For this review, use the dimensioned drawing (mm, ordinates from the lowest corner) and the shaded views. A direction names the side the tool comes from. Coordinates: 2 decimals unless noted, no trailing zeros. Order: outer loops, then holes, each group sorted by start corner. A loop starts at its lowest first (then second) coordinate and runs counter-clockwise, first axis right, second up. Notation, with made-up numbers: M 6.5,13 L 25.5,13 A37 cw 25.5,50 Z; hole C 66.5,-1.5 d5. An arc over 180 degrees is marked long. Answer in a Markdown table with one row per item.
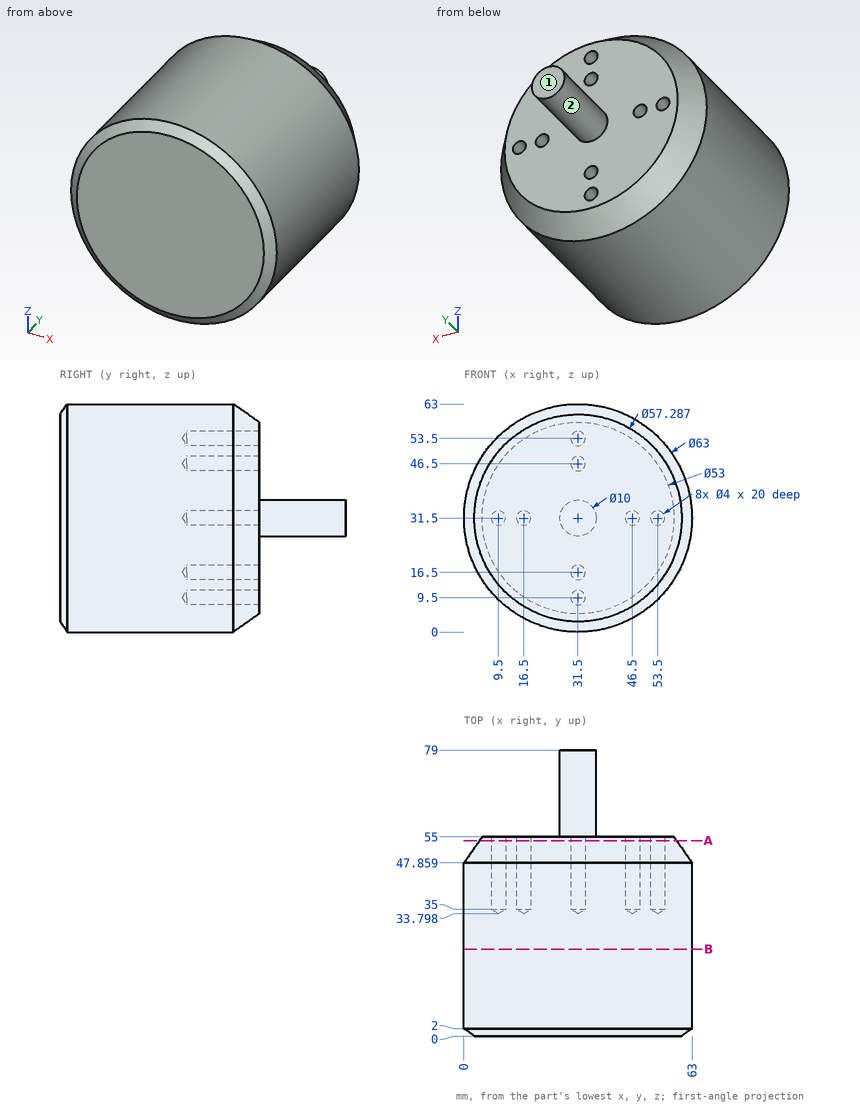
(1) Insertion check: P1, Ø12, axis at x = 24, y = 26.5, coming from the +Z side; P2, Ø1, axis at x = 8.5, y = 35.5, coming from the +Z side (1 decimal); P3, Ø3, axis at x = 45, y = 47, coming from the -Z side (1 decimal). Each pin has a flat end and moves straight along its axis. Give the tip position at first contact, or say it passes through.
Report:
| item | result |
|---|---|
| P1 | z = 62.96 |
| P2 | z = 53.5 |
| P3 | z = 2.4 |
(2) To check wall thickness, follow line 1 (X direction, y = 43, z = 31.5); line 2 (X direction, y = 47, z = 31) (1 decimal). State the ranges of each line that lie inside material, in increasing order. Write a range as [from, to].
Report:
| item | result |
|---|---|
| line 1 | [0, 7.5], [11.5, 14.5], [18.5, 44.5], [48.5, 51.5], [55.5, 63] |
| line 2 | [0, 7.6], [11.4, 14.6], [18.4, 44.6], [48.4, 51.6], [55.4, 63] |
(3) Take a section at B-B (y = 24). Write out the cut boundary in (x, z), then the cut area to 3 significant figures.
Report:
| item | result |
|---|---|
| outline | C 31.5,31.5 d63 |
| area | 3,120 mm^2 |
(4) Machinability: for the marked faces 1 and 2, which of the approach directions +Z, -Z, +X, -X, +Y, -Y give a long, thin tool a straight path to every point of the face, cutting with its end or side? Answer none if there is none.
Report:
| item | result |
|---|---|
| face 1 | +Z, -Z, +X, -X, +Y |
| face 2 | +Y |
(5) Take a section at A-A (y = 54). State how many separate pieces and enclosed holes the cut face has, then the cut area to 3 significant figures.
Report:
| item | result |
|---|---|
| separate pieces | 1 |
| enclosed holes | 8 |
| area | 2,220 mm^2 |
